Design review of the part built by this model. Coordinates are the model's own, in mm. A direction names the side the tool comes from. Round coordinates to 2 decimals unless told otherwise and drop trailing zeros. Loops run counter-clockwise (first coordinate to the right, second up) from the corner with the lowest first, then second, coordinate; pieces in that order, holes last. Notation, with made-up numbers: M 37.25,53 L 72.25,53 A34 ccw 72.25,85 Z; hole C -0.5,37 d7. An arc over 180 degrees is marked long. One line per item, written item: value. Start each with the question number.
Item 1: We need section C-C (y = 0). Write out the cut boundary in (x, z).
Item 2: We need section D-D (y = 6.5). Write out the cut boundary in (x, z).
Item 3: We need section A-A (z = 16). Write out the cut boundary in (x, y).
Item 4: We need section B-B (z = -24). Write out the cut boundary in (x, y), then the cut area to 3 significant figures.
Item 5: Mouldability with a two-part tool opening along Y and no side actions: class faces 1 (the flat face through (1, 10, -8)), 2 (the flat face through (0, 0, -15)), 3 (the cylindrical face through (0.99, 3.43, 14.45)) as released by +Y, released by -Y, zero draft, split by the parting line, or undercut.
Item 6: For line 1 along Y through (x, z) = (1.1, 16); line 2 along Y through (x, z) = (1.6, 7); line 3 along Z through (x, y) = (0.85, -3), list the stretches that pass through material, from the lowest coordinate up.
Item 7: Clearance check with a flat-ended pin moving along its axis: pin 1 (2.5 mm diameter, centred on y = 3.5, z = 16, fed in from -X). State where the tip first meets the part, or that it passes through.
Item 8: For faces 4 (the cylindrical face through (1.014, 6.361, 0.027)), 5 (the flat face through (1, 0, -36)), list the 3-axis set-ups (+Z, -Z, +X, -X, +Y, -Y) from which the entire face can be reached by the end or side of a thin tool; tool diameter is ignored.
from build123d import *

# Parameters (mm, degrees)
SKETCH_1_R      = 1.55
EXTRUDE_1_DEPTH = 2
FILLET_1_R      = 1.01


with BuildPart() as part:
    # 草图1 → 凸台-拉伸1 (new body)
    with BuildSketch(Plane(origin=(0, 0, 0), x_dir=(0, 0, -1), z_dir=(1, 0, 0))):
        Polygon((20, -10), (-20, -10), (-20, 10), (20, 10), (36, 10), (36, -10), align=None)
        with Locations((8, 0)):
            Circle(SKETCH_1_R, mode=Mode.SUBTRACT)
        with Locations((16, 3.5)):
            Circle(SKETCH_1_R, mode=Mode.SUBTRACT)
        with Locations((16, -3.5)):
            Circle(SKETCH_1_R, mode=Mode.SUBTRACT)
        with Locations(Location((-16, -3.5, 0), (0, 0, 180))):
            Circle(SKETCH_1_R, mode=Mode.SUBTRACT)
        with Locations(Location((-16, 3.5, 0), (0, 0, 180))):
            Circle(SKETCH_1_R, mode=Mode.SUBTRACT)
        with Locations((24, 1)):
            Circle(SKETCH_1_R, mode=Mode.SUBTRACT)
        with Locations((32, 1)):
            Circle(SKETCH_1_R, mode=Mode.SUBTRACT)
        Polygon((-12, -5.00684766), (-6.277888388, 0), (-12, 5.00684766), align=None, mode=Mode.SUBTRACT)
        Polygon((-9.722111612, -7), (-4, -1.99315234), (1.722111612, -7), align=None, mode=Mode.SUBTRACT)
        Polygon((-9.722111612, 7), (-4, 1.99315234), (1.722111612, 7), align=None, mode=Mode.SUBTRACT)
        Polygon((4, 5.00684766), (4, -5.00684766), (-1.722111612, 0), align=None, mode=Mode.SUBTRACT)
    extrude(amount=EXTRUDE_1_DEPTH)

    # 圆角1
    fillet_1_edges = [part.edges().sort_by_distance(p)[0] for p in [
        (1, 7, -1.722111612),
        (1, 7, 9.722111612),
        (1, 1.99315234, 4),
        (1, 5.00684766, 12),
        (1, -5.00684766, 12),
        (1, 0, 6.277888388),
        (1, -7, 9.722111612),
        (1, -7, -1.722111612),
        (1, -1.99315234, 4),
        (1, 5.00684766, -4),
        (1, 0, 1.722111612),
        (1, -5.00684766, -4),
    ]]
    fillet(fillet_1_edges, radius=FILLET_1_R)


solid = part.part
A:
1. outline: M 0,-36 L 2,-36 L 2,-33.18 L 0,-33.18 Z; M 0,-30.82 L 2,-30.82 L 2,-25.18 L 0,-25.18 Z; M 0,-22.82 L 2,-22.82 L 2,-9.55 L 0,-9.55 Z; M 0,-6.45 L 2,-6.45 L 2,-4 L 0,-4 Z; M 0,1.2 L 2,1.2 L 2,6.8 L 0,6.8 Z; M 0,12 L 2,12 L 2,20 L 0,20 Z
2. outline: M 0,-36 L 2,-36 L 2,0.09 L 0,0.09 Z; M 0,7.91 L 2,7.91 L 2,20 L 0,20 Z
3. outline: M 0,-10 L 2,-10 L 2,-5.05 L 0,-5.05 Z; M 0,-1.95 L 2,-1.95 L 2,1.95 L 0,1.95 Z; M 0,5.05 L 2,5.05 L 2,10 L 0,10 Z
4. outline: M 0,-10 L 2,-10 L 2,-0.55 L 0,-0.55 Z; M 0,2.55 L 2,2.55 L 2,10 L 0,10 Z
4. area: 33.8 mm2
5. face 1: released by +Y
5. face 2: zero draft
5. face 3: undercut
6. line 1: -10 to -5.05, -1.95 to 1.95, 5.05 to 10
6. line 2: -10 to -7, -4.62 to -0.6, 0.6 to 4.62, 7 to 10
6. line 3: -36 to -17.47, -14.53 to -3.98, -1.71 to 2.85, 5.15 to 9.71, 11.98 to 14.53, 17.47 to 20
7. pin 1: through
8. face 4: +X, -X
8. face 5: -Z, +X, -X, +Y, -Y
